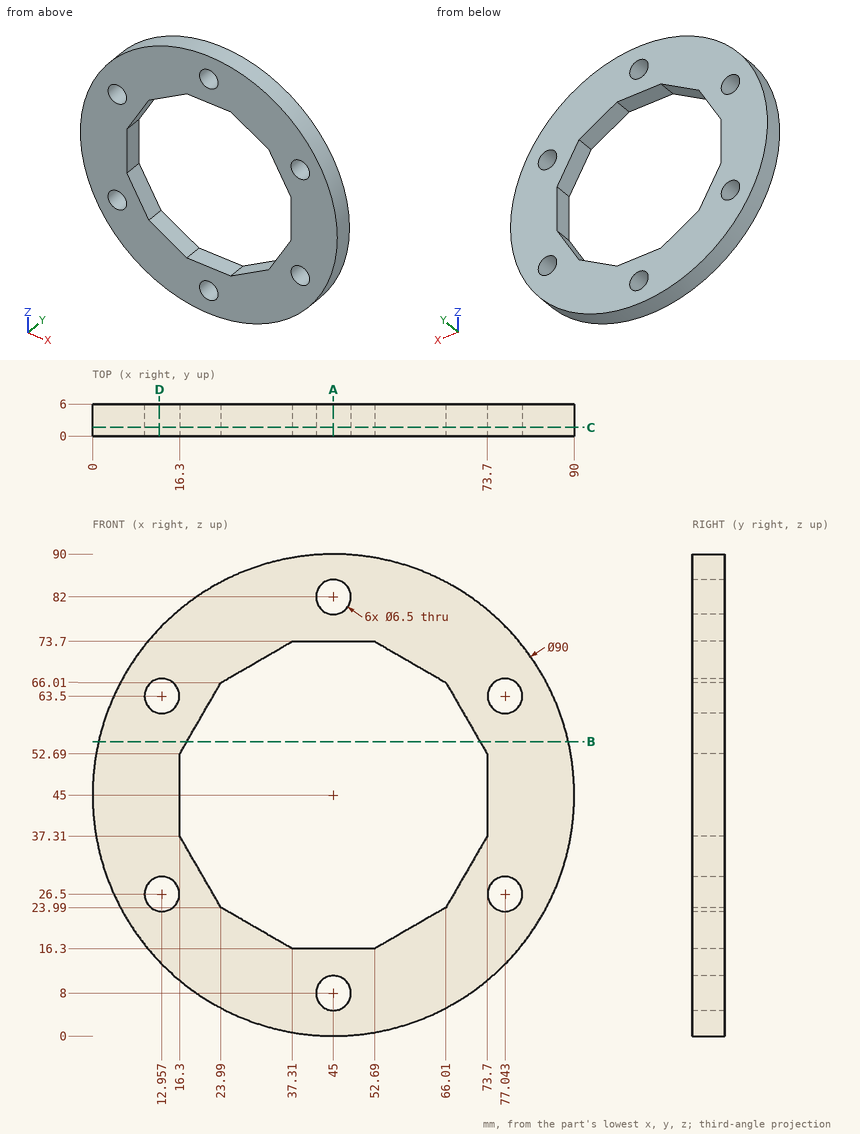
Geometry: see drawing. Coordinates: mm, zero at the bounding-box minimum. Coordinates: 2 decimals unless noted, no trailing zeros. Write each loop counter-clockwise with the first axis right and the second up, starting at its lowest first coordinate (ties: lowest second). Pieces come first, ordered by that corner, then holes. Notation, with made-up numbers: M 73.25,24 L 118.25,24 A17 cw 118.25,48 Z; hole C -38.5,18 d6. An arc over 180 degrees is marked long. Use CSV: the item, a comma, the result in double quotes. Start each with the question number.
1. Cut plane A-A on x = 45. Return the cut outline in (y, z), plus the area to 3 significant figures.
2. Cut plane D-D on x = 12.5. Return the cut outline in (y, z) (1 decimal).
3. First-contact query: P1, Ø1.5, axis at y = 2, z = 57, coming from the +X side; P2, Ø1.8, axis at x = 42, y = 3.5, coming from the +Z side; P3, Ø1.5, axis at y = 4.5, z = 9.5, coming from the +X side. Flat tips, straight axial feed; report the tip coordinate or a pass-through.
4. Ray query, probe 1 along Z at (x, y) = (45, 4.15); probe 2 along Z at (x, y) = (74.5, 5.65); probe 3 along X at (y, z) = (3.95, 25). Return the intervals inside material, ascending.
5. Cut plane B-B on z = 55. Return the cut outline in (x, y) (1 decimal), plus the area to 3 significant figures.
6. Cut plane C-C on y = 1.65. Return the cut outline in (x, z).
Entries:
1,outline,"M 0,0 L 6,0 L 6,4.75 L 0,4.75 Z; M 0,11.25 L 6,11.25 L 6,16.3 L 0,16.3 Z; M 0,73.7 L 6,73.7 L 6,78.75 L 0,78.75 Z; M 0,85.25 L 6,85.25 L 6,90 L 0,90 Z"
1,area,"118 mm²"
2,outline,"M 0,13.9 L 6,13.9 L 6,23.3 L 0,23.3 Z; M 0,29.7 L 6,29.7 L 6,60.3 L 0,60.3 Z; M 0,66.7 L 6,66.7 L 6,76.1 L 0,76.1 Z"
3,P1,"x = 88.57"
3,P2,"z = 89.95"
3,P3,"x = 73.59"
4,probe 1,"0 to 4.75, 11.25 to 16.3, 73.7 to 78.75, 85.25 to 90"
4,probe 2,"11.02 to 24.48, 28.52 to 61.48, 65.52 to 78.98"
4,probe 3,"4.69 to 10.07, 15.84 to 23.41, 66.59 to 74.16, 79.93 to 85.31"
5,outline,"M 1.1,0 L 17.6,0 L 17.6,6 L 1.1,6 Z; M 72.4,0 L 88.9,0 L 88.9,6 L 72.4,6 Z"
5,area,"198 mm²"
6,outline,"C 45,45 d90; hole C 12.96,26.5 d6.5; hole C 12.96,63.5 d6.5; hole M 16.3,37.31 L 23.99,23.99 L 37.31,16.3 L 52.69,16.3 L 66.01,23.99 L 73.7,37.31 L 73.7,52.69 L 66.01,66.01 L 52.69,73.7 L 37.31,73.7 L 23.99,66.01 L 16.3,52.69 Z; hole C 45,8 d6.5; hole C 45,82 d6.5; hole C 77.04,26.5 d6.5; hole C 77.04,63.5 d6.5"
